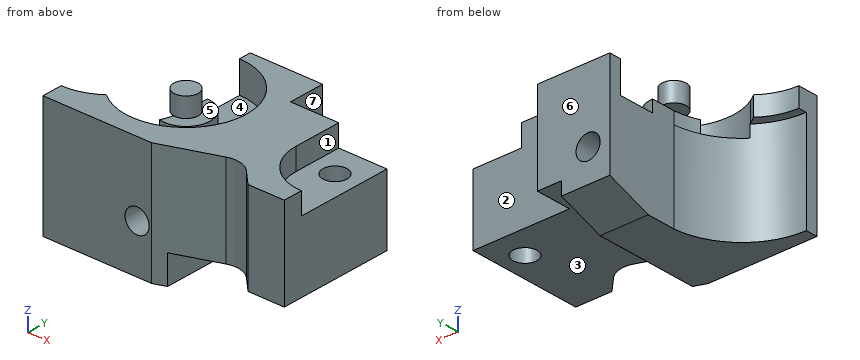
```python
from build123d import *

# Parameters (mm, degrees)
BOSS_EXTRUDE2_DEPTH      = 50
SKETCH2_R                = 5
CUT_EXTRUDE1_DEPTH       = 78.409624725
SKETCH2_5_R              = 5
CUT_EXTRUDE2_DEPTH       = 9
CUT_EXTRUDE12_DEPTH      = 78.409624725
CUT_EXTRUDE12_DEPTH_BACK = 42
CUT_EXTRUDE14_DEPTH      = 42
CUT_EXTRUDE16_DEPTH      = 78.409624725
CUT_EXTRUDE16_DEPTH_BACK = 78.409624725
SKETCH41_R               = 25
CUT_EXTRUDE17_DEPTH      = 13
BOSS_EXTRUDE8_START      = 5
BOSS_EXTRUDE8_DEPTH      = 5
SKETCH43_R               = 5
BOSS_EXTRUDE9_DEPTH      = 8
CUT_EXTRUDE19_DEPTH      = 92.609224426
CUT_EXTRUDE21_DEPTH      = 86.463442477
CUT_EXTRUDE21_DEPTH_BACK = 86.463442477
SKETCH45_W               = 50
SKETCH45_H               = 12
SKETCH46_R               = 5
CUT_EXTRUDE22_DEPTH      = 95.704804524


with BuildPart() as part:
    # Sketch1 → Boss-Extrude2 (new body)
    with BuildSketch(Plane.XY):
        with BuildLine():
            Line((10, 16.5), (10, 31.5))
            Line((10, 31.5), (-50, 31.5))
            Line((-50, 31.5), (-50, -31.5))
            Line((-50, -31.5), (-5, -31.5))
            Line((-5, -31.5), (18.339650933, -23.005061782))
            ThreePointArc((18.339650933, -23.005061782), (23.924248506, -22.639027919), (28.830920178, -25.330920178))
            Line((28.830920178, -25.330920178), (35, -31.5))
            Line((35, -31.5), (50, -31.5))
            Line((50, -31.5), (50, 16.5))
            Line((50, 16.5), (10, 16.5))
        make_face()
    extrude(amount=BOSS_EXTRUDE2_DEPTH)

    # Sketch2 → Cut-Extrude1 (cut, through all)
    with BuildSketch(Plane.XY.offset(50)):
        with Locations((40, 3.5)):
            Circle(SKETCH2_R)
    extrude(amount=-CUT_EXTRUDE1_DEPTH, mode=Mode.SUBTRACT)

    # Sketch2<5> → Cut-Extrude2 (cut)
    with BuildSketch(Plane.XY.offset(50)):
        with BuildLine():
            Line((50, 16.5), (30, 16.5))
            Line((30, 16.5), (30, -3.523038751))
            ThreePointArc((30, -3.523038751), (35.857864376, -17.665174375), (50, -23.523038751))
            Line((50, -23.523038751), (50, 16.5))
        make_face()
        with Locations((40, 3.5)):
            Circle(SKETCH2_5_R, mode=Mode.SUBTRACT)
    extrude(amount=-CUT_EXTRUDE2_DEPTH, mode=Mode.SUBTRACT)

    # Sketch30 → Cut-Extrude12 (cut, two sides: drawn at the far end of the back side and taken through both)
    with BuildSketch(Plane(origin=(0, 0, 0), x_dir=(-1, 0, 0), z_dir=(0, 0, -1)).offset(-CUT_EXTRUDE12_DEPTH_BACK)):
        with BuildLine():
            Line((291.204939457, -25.963430676), (50, -26.5))
            ThreePointArc((50, -26.5), (29.463716543, -18.431732275), (20, 1.5))
            Line((20, 1.5), (20, 31.5))
            Line((20, 31.5), (20, 272.705536266))
            Line((20, 272.705536266), (377.141103264, 597.005821897))
            Line((377.141103264, 597.005821897), (648.346042721, 298.336854955))
            Line((648.346042721, 298.336854955), (291.204939457, -25.963430676))
        make_face()
    extrude(amount=CUT_EXTRUDE12_DEPTH + CUT_EXTRUDE12_DEPTH_BACK, mode=Mode.SUBTRACT)

    # Sketch15 → Cut-Extrude14 (cut)
    with BuildSketch(Plane.XY.offset(50)):
        with BuildLine():
            Line((-20, 1.5), (-20, 26.5))
            ThreePointArc((-20, 26.5), (-44.154267569, 7.947585455), (-32.45893634, -20.174291344))
            ThreePointArc((-32.45893634, -20.174291344), (-23.864179013, -10.696774301), (-20, 1.5))
        make_face()
    extrude(amount=-CUT_EXTRUDE14_DEPTH, mode=Mode.SUBTRACT)

    # Sketch39 → Cut-Extrude16 (cut, two sides: drawn at the far end of the back side and taken through both)
    with BuildSketch(Plane.XY.offset(50).offset(-CUT_EXTRUDE16_DEPTH_BACK)):
        with BuildLine():
            Line((-50, 31.5), (-50, -23))
            ThreePointArc((-50, -23), (-42.405705612, -21.710059713), (-35.66325351, -17.984929805))
            ThreePointArc((-35.66325351, -17.984929805), (-43.580958898, 9.802913792), (-20, 26.5))
            Line((-20, 26.5), (-20, 31.5))
            Line((-20, 31.5), (-50, 31.5))
        make_face()
    extrude(amount=CUT_EXTRUDE16_DEPTH + CUT_EXTRUDE16_DEPTH_BACK, mode=Mode.SUBTRACT)

    # Sketch41 → Cut-Extrude17 (cut)
    with BuildSketch(Plane.XY.offset(50)):
        with Locations((-20, 1.5)):
            Circle(SKETCH41_R)
    extrude(amount=-CUT_EXTRUDE17_DEPTH, mode=Mode.SUBTRACT)

    # Sketch42 → Boss-Extrude8 (add)
    with BuildSketch(Plane.XY.offset(37).offset(BOSS_EXTRUDE8_START)):
        with BuildLine():
            Line((-20, 11.5), (-20, 1.5))
            ThreePointArc((-20, 1.5), (-20.751988631, -3.460904975), (-22.320276916, -8.227091808))
            ThreePointArc((-22.320276916, -8.227091808), (-10.068461396, 0.331864322), (-20, 11.5))
        make_face()
    extrude(amount=-BOSS_EXTRUDE8_DEPTH)

    # Sketch43 → Boss-Extrude9 (add)
    with BuildSketch(Plane.XY.offset(42)):
        with Locations(Location((-20, 1.5, 0), (0, 0, 261.397396505))):
            Circle(SKETCH43_R)
    extrude(amount=BOSS_EXTRUDE9_DEPTH)

    # Sketch44 → Cut-Extrude19 (cut, through all)
    with BuildSketch(Plane.ZY.offset(20)):
        Polygon((0, 13.5), (6.551464217, 31.5), (0, 31.5), align=None)
    extrude(amount=-CUT_EXTRUDE19_DEPTH, mode=Mode.SUBTRACT)

    # Sketch45 → Cut-Extrude21 (cut, two sides: drawn at the far end of the back side and taken through both)
    with BuildSketch(Plane(origin=(0, 16.5, 0), x_dir=(1, 0, 0), z_dir=(0, 1, 0)).offset(-CUT_EXTRUDE21_DEPTH_BACK)):
        with Locations((25, -6)):
            Rectangle(SKETCH45_W, SKETCH45_H)
    extrude(amount=CUT_EXTRUDE21_DEPTH + CUT_EXTRUDE21_DEPTH_BACK, mode=Mode.SUBTRACT)

    # Sketch46 → Cut-Extrude22 (cut, through all)
    with BuildSketch(Plane(origin=(0, 31.5, 0), x_dir=(1, 0, 0), z_dir=(0, 1, 0))):
        with Locations(Location((-11, -20, 0), (0, 0, 180))):
            Circle(SKETCH46_R)
    extrude(amount=-CUT_EXTRUDE22_DEPTH, mode=Mode.SUBTRACT)


solid = part.part
```
Check sheet for the modelled part. Datum: model origin and axes. Units: mm. Face numbers are marked on the shaded views. A direction names the side the tool comes from. Give positions to 0.01 mm unless a question says otherwise; leave off trailing zeros. Loops run counter-clockwise (first coordinate to the right, second up) from the corner with the lowest first, then second, coordinate; pieces in that order, holes last. Notation, with made-up numbers: M -22.5,-23 L 11.5,-23 A33 cw 11.5,16 Z; hole C 34.25,0.25 d8. An arc over 180 degrees is marked long. Answer as CSV lines item,"result".
Item 1: Scan lines: L1, parallel to Y at x = 40, z = 20; L2, parallel to X at y = 2, z = 38.5 (1 decimal); L3, parallel to Z at x = -18, y = -19.5. Record each from-to range of solid material in increasing order.
Reply:
L1,"-31.5 to -1.5, 8.5 to 16.5"
L2,"-20 to -10, 5 to 35.2, 44.8 to 50"
L3,"0 to 37"
Item 2: Draft check along X on the marked faces 5, 6 and 7. Enter one of: pulls with the +X half, pulls with the -X half, needs draft (parallel to the pull), parting line crosses it, or undercut.
Reply:
face 5,"undercut"
face 6,"needs draft"
face 7,"pulls with the +X half"
Item 3: Sectioned sample at C-C, the plane z = 31. Enter the section's corners in (x, y).
Reply:
outline,"M -50,-31.5 L -5,-31.5 L 18.34,-23.01 A10 cw 28.83,-25.33 L 35,-31.5 L 50,-31.5 L 50,16.5 L 10,16.5 L 10,31.5 L -20,31.5 L -20,1.5 A30 cw -50,-26.5 Z; hole C 40,3.5 d10"
Item 4: Sectioned sample at A-A, the plane z = 20. Enter the section's corners in (x, y).
Reply:
outline,"M -50,-31.5 L -16,-31.5 L -16,31.5 L -20,31.5 L -20,1.5 A30 cw -50,-26.5 Z; M -6,-31.5 L -5,-31.5 L 18.34,-23.01 A10 cw 28.83,-25.33 L 35,-31.5 L 50,-31.5 L 50,16.5 L 10,16.5 L 10,31.5 L -6,31.5 Z; hole C 40,3.5 d10"
Item 5: Sectioned sample at D-D, the plane x = 3. Enter the section's corners in (y, z), then the cut area to 3 significant figures.
Reply:
outline,"M -28.59,12 L 31.5,12 L 31.5,50 L 11.3,50 L 11.3,37 L -8.3,37 L -8.3,50 L -28.59,50 Z"
area,"2,030 mm^2"
Item 6: Sectioned sample at B-B, the plane y = 3.5. Enter the section's corners in (x, z), then the cut area to 3 significant figures.
Reply:
outline,"M -24.58,42 L -20,42 L -20,0 L 0,0 L 0,12 L 35,12 L 35,41 L 30,41 L 30,50 L 4.92,50 L 4.92,37 L -10.2,37 L -10.2,42 L -15.42,42 L -15.42,50 L -24.58,50 Z; M 45,12 L 50,12 L 50,41 L 45,41 Z; hole C -11,20 d10"
area,"2,150 mm^2"
Item 7: Depth check by flat-ended pin: pin 1 Ø10 at (x, y) = (38.5, -8.5) entering from +Z; pin 2 Ø6 at (y, z) = (9, 21.5) entering from -X; pin 3 Ø2.5 at (x, y) = (-40.5, -20) entering from -Z. Enter the tip coordinate at first touch or a pass-through.
Reply:
pin 1,"z = 41"
pin 2,"x = -20"
pin 3,"z = 42"
Item 8: Set-up check for the marked faces 1, 2, 3 and 4: record each of +Z, -Z, +X, -X, +Y, -Y from which the full face is reachable in a straight line by a thin tool's end or side.
Reply:
face 1,"+Z, +X, +Y"
face 2,"+Z, -Z, +X, +Y"
face 3,"-Z, +X, +Y, -Y"
face 4,"+Z"
